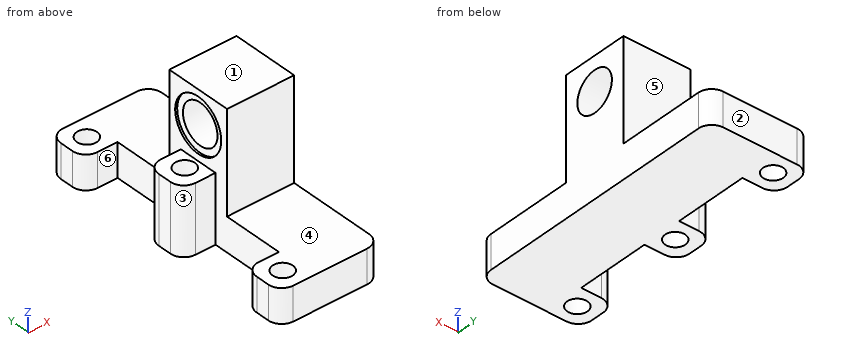
Autodesk Inventor part; units mm, degrees
ref_plane "YZ Plane" through (0, 0, 0) normal (1, 0, 0) x (0, 1, 0)
ref_plane "XZ Plane" through (0, 0, 0) normal (0, 1, 0) x (-1, 0, 0)
sketch "Sketch1" plane through (0, 0, 0) normal (0, 1, 0) x (-1, 0, 0)
  line L0 (0, 0) -> (10, 0)
  line L1 (10, 0) -> (10, -10)
  line L2 (10, -10) -> (0, -10)
  line L3 (0, -10) -> (0, 0)
  dimension "d0" = 10
  dimension "d1" = 10
extrude "Extrusion1" add sketch "Sketch1" along normal blind 40
sketch "Sketch2" plane through (-10, 0, -10) normal (-1, 0, 0) x (0, 0, 1)
  line L0 (0, 40) -> (10, 40)
  line L1 (10, 40) -> (0, 40)
  line L2 (0, 40) -> (0, 34)
  line L3 (0, 34) -> (10, 34)
  line L4 (10, 34) -> (10, 40)
  point P0 (10, 0)
  dimension "d4" = 10
  dimension "d5" = 6
extrude "Extrusion2" add sketch "Sketch2" along normal blind 5
sketch "Sketch3" plane through (-10, 0, -10) normal (-1, 0, 0) x (0, 0, 1)
  line L0 (10, 0) -> (10, 40)
  line L1 (10, 0) -> (0, 0)
  line L2 (0, 0) -> (0, 6)
  line L3 (0, 6) -> (10, 6)
  line L4 (10, 6) -> (10, 0)
  dimension "d8" = 10
  dimension "d9" = 6
extrude "Extrusion3" add sketch "Sketch3" along normal blind 5
sketch "Sketch4" plane through (-10, 34, -10) normal (-1, 0, 0) x (0, 0, 1)
  line L0 (10, -34) -> (10, 6)
  line L1 (10, -34) -> (10, -14)
  line L2 (10, -14) -> (10, -17)
  line L3 (10, -17) -> (0, -17)
  line L4 (0, -17) -> (0, -11)
  line L5 (0, -11) -> (10, -11)
  line L6 (10, -11) -> (10, -17)
  point P0 (10, -11)
  dimension "d12" = 20
  dimension "d13" = 3
  dimension "d14" = 10
  dimension "d15" = 6
extrude "Extrusion4" add sketch "Sketch4" along normal blind 5
sketch "Sketch5" plane through (0, 0, 0) normal (0, 0, 1) x (1, 0, 0)
  line L0 (-15, 0) -> (-15, 6)
  line L1 (-15, 3) -> (-12, 3)
  line L2 (-15, 23) -> (-15, 17)
  line L3 (-15, 20) -> (-12, 20)
  line L4 (-15, 34) -> (-15, 40)
  line L5 (-15, 37) -> (-12, 37)
  point P0 (0, 0)
  dimension "d18" = 3
  dimension "d19" = 3
  dimension "d20" = 3
hole "Hole1" at (-12, 37, 0) at (-12, 20, 0) at (-12, 3, 0) direction (0, 0, -1) diameter 3 end through all
fillet "Fillet1" radius 2 8 edges at (-15, 17, -5) (-15, 23, -5) (-15, 40, -5) (-15, 34, -5) (-15, 6, -5) (-15, 0, -5) (0, 40, -5) (0, 0, -5)
sketch "Sketch6" plane through (0, 2, -10) normal (1, 0, 0) x (0, 0, -1)
  point P0 (-10, -2)
sketch "Sketch7" plane through (0, 0, 0) normal (0, 0, 1) x (1, 0, 0)
  point P0 (0, 0)
ref_plane "Work Plane1" through (0, 0, -5) normal (0, 0, 1) x (1, 0, 0)
sketch "Sketch10" plane through (0, 0, -5) normal (0, 0, 1) x (1, 0, 0)
  point P0 (0, 0)
sketch "Sketch12" plane through (-10, 23, 0) normal (0, 0, 1) x (1, 0, 0)
  line L0 (10, -23) -> (10, -3)
  line L1 (10, -23) -> (30, -23) construction
  line L2 (10, -3) -> (10, 2)
  line L3 (0, 0) -> (0, 11)
  line L4 (10, 2) -> (0, 2)
  line L5 (0, 2) -> (0, -8)
  line L6 (0, -8) -> (10, -8)
  line L7 (10, -8) -> (10, 2)
  dimension "d45" = 20
  dimension "d46" = 90
  dimension "d47" = 5
  dimension "d48" = 10
  dimension "d49" = 10
extrude "Extrusion6" add sketch "Sketch12" along normal blind 10
sketch "Sketch13" plane through (0, 2, -10) normal (1, 0, 0) x (0, 0, -1)
  line L0 (-10, 13) -> (-20, 13)
  line L1 (-18, 13) -> (-18, 18)
  line L2 (-18, 23) -> (-18, 13)
  line L3 (-18, 18) -> (-15, 18)
  circle A0 centre (-15, 18) radius 3
  point P0 (-10, -2)
  point P1 (-12, 13)
  dimension "d54" = 5
  dimension "d55" = 3
  dimension "d56" = 6
extrude "Extrusion7" cut sketch "Sketch13" against normal blind 10
sketch "Sketch14" plane through (0, 2, -10) normal (1, 0, 0) x (0, 0, -1)
  arc A0 (-10, 11) -> (-12, 13) centre (-12, 11) ccw
  line L0 (-12, 13) -> (-5, 13)
  line L1 (-5, 13) -> (-5, -2)
  line L2 (0, -2) -> (-10, -2)
  line L3 (-5, -2) -> (-5, 38)
  line L4 (-10, 38) -> (0, 38)
  line L5 (-5, -2) -> (-12, -2)
  line L6 (-12, -2) -> (-12, 13)
  line L7 (-12, 13) -> (-5, 13)
  line L8 (-5, 13) -> (-5, -2)
  arc A1 (-12, 23) -> (-10, 25) centre (-12, 25) ccw
  line L9 (-5, 38) -> (-12, 38)
  line L10 (-12, 38) -> (-12, 23)
  line L11 (-12, 23) -> (-5, 23)
  line L12 (-5, 23) -> (-5, 38)
  dimension "d59" = 7
extrude "Extrusion8" cut sketch "Sketch14" against normal blind 30
sketch "Sketch15" plane through (-10, 23, -10) normal (-1, 0, 0) x (0, 0, 1)
  circle A0 centre (15, -3) radius 3
  circle A1 centre (15, -3) radius 4
  point P0 (10, -23)
  dimension "d62" = 8
extrude "Extrusion9" cut sketch "Sketch15" against normal blind 0.3
properties part number "STUURAS"
Input: part model. Units: mm. Frame: model coordinates. Face numbers are marked on the shaded views. A direction names the side the tool comes from. Give positions to 0.01 mm unless a question says otherwise; leave off trailing zeros. Order: outer loops, then holes, each group sorted by start corner. A loop starts at its lowest first (then second) coordinate and runs counter-clockwise, first axis right, second up.
1. Section C-C on y = 3. Return the cut outline in (x, z).
Derived:
outline: (-15, -10) - (-13.5, -10) - (-13.5, -5) - (-15, -5) - close; (-10.5, -10) - (0, -10) - (0, -5) - (-10.5, -5) - close
2. Material intervals for L1, parallel to Y at x = -12, z = -7.25; L2, parallel to X at y = 20, z = -4; L3, parallel to Y at x = -3, z = 5, sorted ascending.
Derived:
L1: y = 0 to 1.5, 4.5 to 6, 17 to 18.5, 21.5 to 23, 34 to 35.5, 38.5 to 40
L2: x = -15 to -13.5, -10.5 to 0
L3: y = 15 to 17, 23 to 25
3. Mould query, pull axis Y, two halves, no side actions, for the marked faces 1, 2 and 3. Classes: released by +Y, released by -Y, zero draft, split by the parting line, or undercut.
Derived:
face 1: zero draft
face 2: released by +Y
face 3: undercut
4. Pin query (flat end, axial travel): pin 1 (6.5 mm diameter, centred on y = 18.5, z = 5.5, fed in from -X); pin 2 (2.5 mm diameter, centred on x = -12, y = 20, fed in from +Z); pin 3 (3 mm diameter, centred on x = -7, z = -1, fed in from -Y); pin 4 (7 mm diameter, centred on y = 20, z = 5, fed in from -X). Return the tip coordinate at first contact, or that it passes through.
Derived:
pin 1: stops at x = -10
pin 2: passes through
pin 3: stops at y = 15
pin 4: stops at x = -9.7
5. Section D-D on x = -2.5. Return the cut outline in (y, z), and give its area (3 significant figures).
Derived:
outline: (0, -10) - (40, -10) - (40, -5) - (25, -5) - (25, 10) - (15, 10) - (15, -5) - (0, -5) - close; hole circle Ø6 at (20, 5)
area: 322 mm2
6. Section A-A on x = -12. Return the cut outline in (y, z).
Derived:
outline: (0, -10) - (1.5, -10) - (1.5, -5) - (0, -5) - close; (4.5, -10) - (6, -10) - (6, -5) - (4.5, -5) - close; (17, -10) - (18.5, -10) - (18.5, 0) - (17, 0) - close; (21.5, -10) - (23, -10) - (23, 0) - (21.5, 0) - close; (34, -10) - (35.5, -10) - (35.5, -5) - (34, -5) - close; (38.5, -10) - (40, -10) - (40, -5) - (38.5, -5) - close
7. Section B-B on z = 5. Return the cut outline in (x, y).
Derived:
outline: (-10, 15) - (0, 15) - (0, 17) - (-9.7, 17) - (-9.7, 16) - (-10, 16) - close; (-10, 24) - (-9.7, 24) - (-9.7, 23) - (0, 23) - (0, 25) - (-10, 25) - close
8. Reachability of the marked faces 4, 5 and 6 from +Z, -Z, +X, -X, +Y, -Y: full face, straight path, thin tool, end or side. Return the list, or none.
Derived:
face 4: +Z, +X, -X, -Y
face 5: +Z, +X, -X, +Y
face 6: +Z, -Z, -X
